Can you work these out from the drawing? Everything is in mm from the part's minimum corner. A direction names the side the tool comes from. Coordinates: 2 decimals unless noted, no trailing zeros. Order: outer loops, then holes, each group sorted by start corner. A loop starts at its lowest first (then second) coordinate and runs counter-clockwise, first axis right, second up. Notation, with made-up numbers: (83, 81) -> (124, 81) arc R23 cw to (124, 112) -> close; hole circle Ø7 at (13, 28). An arc over 180 degrees is marked (long way). Put each result on its own line as item: value. Start each with the question number.
Q1. We'd pull the mould along Z, two halves only. Please class the marked faces 4, 5 and 6: +Z half, -Z half, draft (parallel to the pull), parting line (faces both ways), or undercut.
Q2. If we section it at C-C (z = 1.25): Please give me the cut outline in (x, y).
Q3. For the marked faces 1, 2 and 3, which set-ups out of +Z, -Z, +X, -X, +Y, -Y let a thin tool reach every point of the face, with its end or its side?
Q4. If we section it at A-A (z = 5): Please give me the cut outline in (x, y).
Q5. Please list where these lines run through material, in increasing order: line 1 along X through (y, z) = (3.7, 5); line 2 along Z through (x, y) = (3, 0.25); line 3 along X through (y, z) = (4.05, 1.5).
Q6. Will these pins go through, and if not, where does the flat tip stop? pin 1 (0.8 mm diameter, centred on y = 4, z = 5, fed in from +X); pin 2 (1.6 mm diameter, centred on y = 1.5, z = 4.5, fed in from -X); pin 3 (1.4 mm diameter, centred on x = 1, z = 4, fed in from +Y).
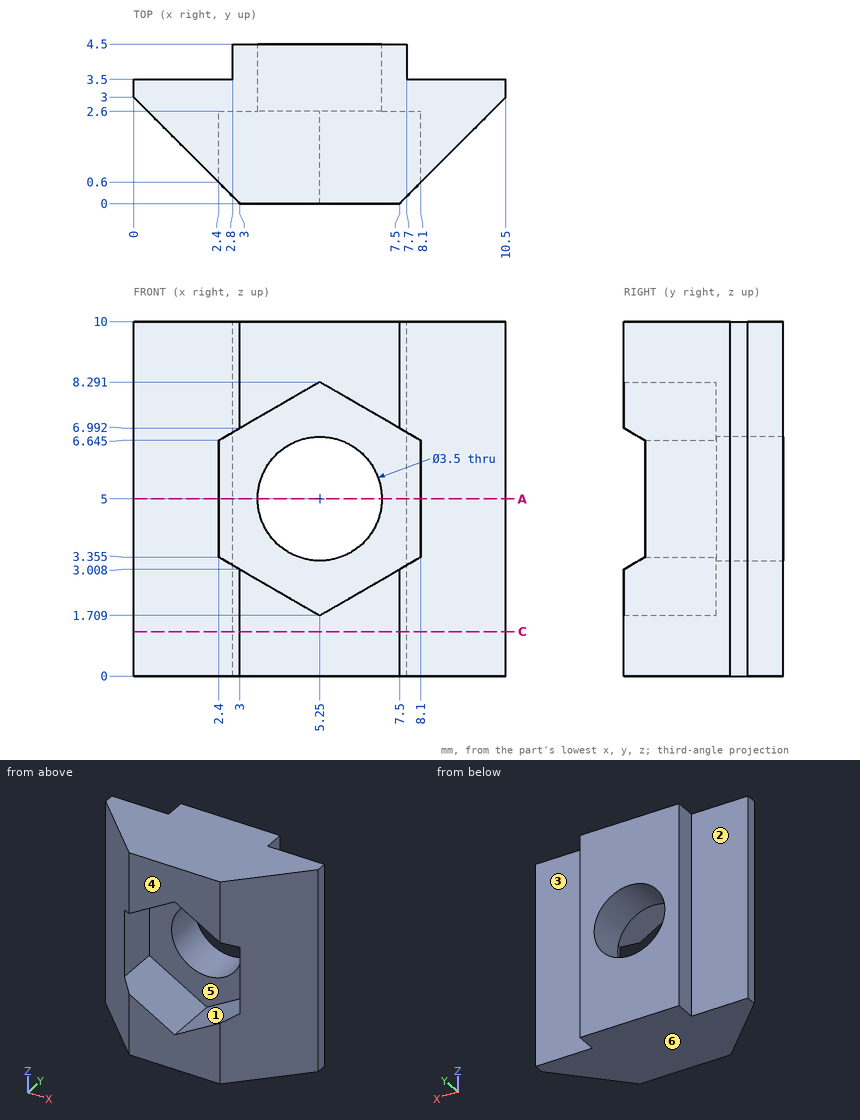
The answers:
1. face 4: draft
1. face 5: undercut
1. face 6: -Z half
2. outline: (0, 3) -> (3, 0) -> (7.5, 0) -> (10.5, 3) -> (10.5, 3.5) -> (7.7, 3.5) -> (7.7, 4.5) -> (2.8, 4.5) -> (2.8, 3.5) -> (0, 3.5) -> close
3. face 1: -Y
3. face 2: +Z, -Z, -X, +Y
3. face 3: +Z, -Z, +X, +Y
4. outline: (0, 3) -> (2.4, 0.6) -> (2.4, 2.6) -> (3.5, 2.6) -> (3.5, 4.5) -> (2.8, 4.5) -> (2.8, 3.5) -> (0, 3.5) -> close; (7, 2.6) -> (8.1, 2.6) -> (8.1, 0.6) -> (10.5, 3) -> (10.5, 3.5) -> (7.7, 3.5) -> (7.7, 4.5) -> (7, 4.5) -> close
5. line 1: 2.8 to 3.5, 7 to 7.7
5. line 2: 0 to 3.01, 6.99 to 10
5. line 3: 2.8 to 7.7
6. pin 1: x = 7.7
6. pin 2: x = 0.7
6. pin 3: y = 3.5
